Source: three-view drawing plus pictorial views. Frame: mm from the lowest corner of the part. A direction names the side the tool comes from. Give positions to 0.01 mm unless a question says otherwise; leave off trailing zeros. Order: outer loops, then holes, each group sorted by start corner. A loop starts at its lowest first (then second) coordinate and runs counter-clockwise, first axis right, second up. Notation, with made-up numbers: (-28, 70.25) - (1, 70.25) arc R25 cw to (1, 99.25) - close; hole circle Ø7 at (52.25, 47.25). An arc over 180 degrees is marked (long way). Answer in a Markdown table with one row per item. Add a question column.
1. Contact query for flat-ended pins moving along their axis: pin 1 (7.5 mm diameter, centred on y = 15.5, z = 4.5, fed in from -X); pin 2 (2.5 mm diameter, centred on y = 18.5, z = 2, fed in from +X); pin 3 (5 mm diameter, centred on x = 7.5, y = 35, fed in from +Z). Output: stop coordinate, or through.
2. Ray query, line 1 (Z direction, x = 106.5, y = 39); line 2 (Z direction, x = 98, y = 1.9); line 3 (X direction, y = 1, z = 4). Return the intervals inside material, ascending. Write a range as [from, to].
3. Section query D-D on z = 37.5. Return loops of the section in (x, y).
4. Section query B-B on x = 41.5. Return loops of the section in (y, z).
5. Access query for the marked faces 4 and 5. Directions: +Z, -Z, +X, -X, +Y, -Y. A direction counts if a zero-diameter tool reaches every point of the face in a straight line with its end or side. Return the directions, or none.
6. Section query A-A on z = 62. Return loops of the section in (x, y) (3 decimals), and give its area (3 significant figures).
7. Mould query, pull axis X, two halves, no side actions, for the marked faces 1, 2 and 3. Classes: released by +X, released by -X, zero draft, split by the parting line, or undercut.
8. Section query C-C on y = 29. Return loops of the section in (x, z).
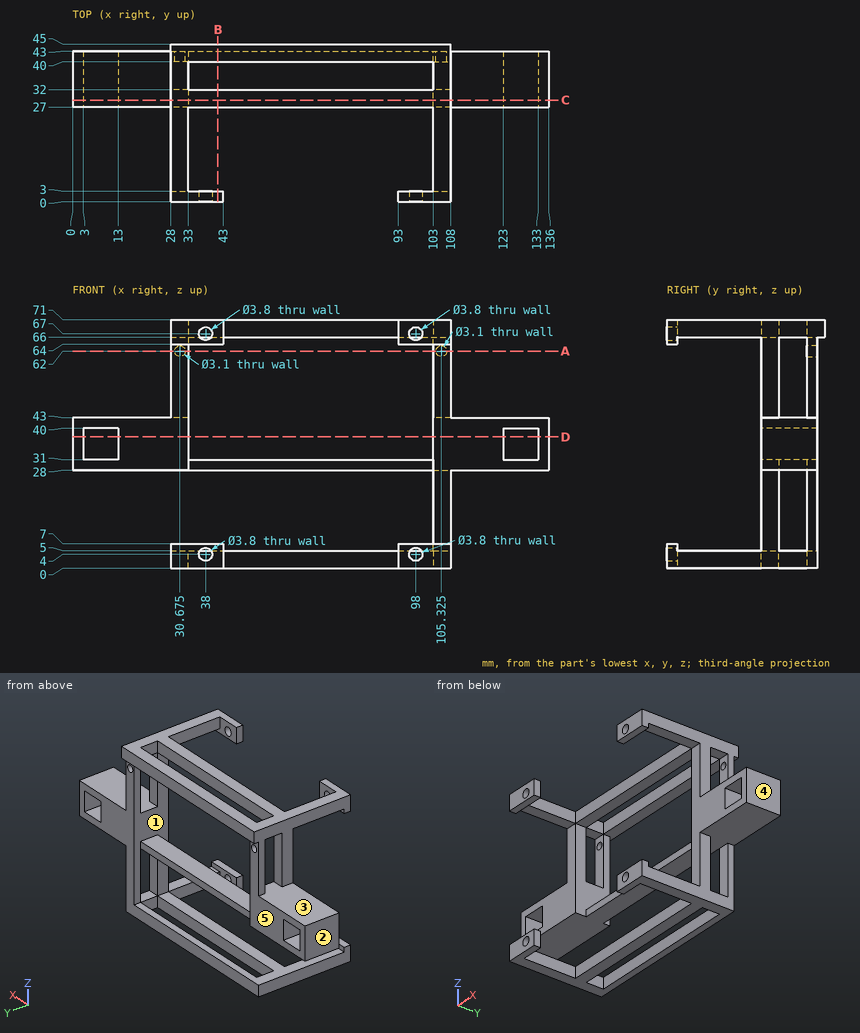
Answer:
| question | item | result |
|---|---|---|
| 1 | pin 1 | stops at x = 28 |
| 1 | pin 2 | stops at x = 108 |
| 1 | pin 3 | stops at z = 43 |
| 2 | line 1 | z = [0, 5], [28, 43], [66, 71] |
| 2 | line 2 | z = [0, 2.1], [5.9, 7], [64, 65.1], [68.9, 71] |
| 2 | line 3 | x = [28, 36.1], [39.9, 43], [93, 96.1], [99.9, 108] |
| 3 | outline | (0, 27) - (3, 27) - (3, 43) - (0, 43) - close; (13, 27) - (33, 27) - (33, 43) - (13, 43) - close; (103, 27) - (123, 27) - (123, 43) - (103, 43) - close; (133, 27) - (136, 27) - (136, 43) - (133, 43) - close |
| 4 | outline | (0, 0) - (3, 0) - (3, 7) - (0, 7) - close; (0, 64) - (3, 64) - (3, 71) - (0, 71) - close; (27, 0) - (32, 0) - (32, 5) - (27, 5) - close; (27, 66) - (32, 66) - (32, 71) - (27, 71) - close; (32, 28) - (40, 28) - (40, 31) - (32, 31) - close; (40, 0) - (43, 0) - (43, 5) - (40, 5) - close; (40, 66) - (45, 66) - (45, 71) - (40, 71) - close |
| 5 | face 4 | +Z, -Z, +X, +Y, -Y |
| 5 | face 5 | -Z, +X, -X, +Y |
| 6 | outline | (28, 27) - (33, 27) - (33, 32) - (28, 32) - close; (28, 40) - (29.125, 40) - (29.125, 43) - (28, 43) - close; (32.225, 40) - (33, 40) - (33, 43) - (32.225, 43) - close; (103, 27) - (108, 27) - (108, 32) - (103, 32) - close; (103, 40) - (103.775, 40) - (103.775, 43) - (103, 43) - close; (106.875, 40) - (108, 40) - (108, 43) - (106.875, 43) - close |
| 6 | area | 61.4 mm² |
| 7 | face 1 | undercut |
| 7 | face 2 | released by -X |
| 7 | face 3 | zero draft |
| 8 | outline | (0, 28) - (33, 28) - (33, 66) - (103, 66) - (103, 5) - (28, 5) - (28, 0) - (108, 0) - (108, 28) - (136, 28) - (136, 43) - (108, 43) - (108, 71) - (28, 71) - (28, 43) - (0, 43) - close; hole (3, 31) - (13, 31) - (13, 40) - (3, 40) - close; hole (123, 31) - (133, 31) - (133, 40) - (123, 40) - close |
